Part print with two shaded views. Sizes in mm from the minimum x, y, z corner. Round coordinates to 2 decimals unless told otherwise and drop trailing zeros. Loops run counter-clockwise (first coordinate to the right, second up) from the corner with the lowest first, then second, coordinate; pieces in that order, holes last. Notation, with made-up numbers: (20, 15.5) -> (36, 15.5) arc R15 ccw to (36, 35.5) -> close; hole circle Ø8 at (51.5, 39). An arc over 180 degrees is marked (long way). Answer as a JSON object with one key per item and string values. Group by question number.
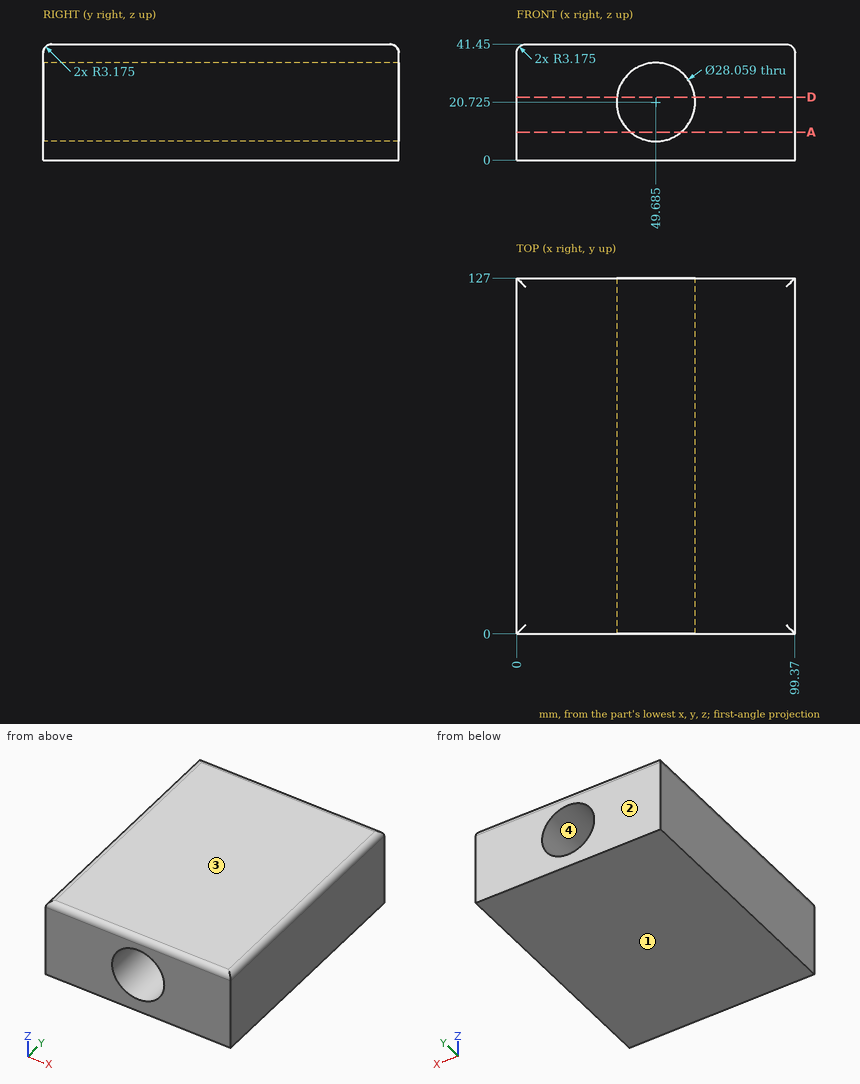
Item 1: Drill centre lines: line 1 (Z direction, x = 49.5, y = 44.5); line 2 (X direction, y = 7.5, z = 20.5); line 3 (X direction, y = 53, z = 29) (1 decimal). Where is each one in solid material? Low to high.
Item 2: Two-plate mould, pull along Z, no slides. Class the marked faces 1, 2, 3 and 4: pulls with the +Z half, pulls with the -Z half, needs draft (parallel to the pull), parting line crosses it, or undercut.
Item 3: Band-saw the part on D-D, the plane z = 22.5. List the corners of the cut face in (x, y).
Item 4: Band-saw the part on A-A, the plane z = 10. List the corners of the cut face in (x, y).
Entries:
{
 "1": {"line 1": "0 to 6.7, 34.75 to 41.45", "line 2": "0 to 35.66, 63.71 to 99.37", "line 3": "0 to 38.4, 61 to 99.4"},
 "2": {"face 1": "pulls with the -Z half", "face 2": "needs draft", "face 3": "pulls with the +Z half", "face 4": "undercut"},
 "3": {"outline": "(0, 0) -> (35.77, 0) -> (35.77, 127) -> (0, 127) -> close; (63.6, 0) -> (99.37, 0) -> (99.37, 127) -> (63.6, 127) -> close"},
 "4": {"outline": "(0, 0) -> (40.64, 0) -> (40.64, 127) -> (0, 127) -> close; (58.73, 0) -> (99.37, 0) -> (99.37, 127) -> (58.73, 127) -> close"}
}
